```python
from build123d import *

# Parameters (mm, degrees)
BOSS_EXTRUDE1_DEPTH        = 19
F_20_0MM_DOWEL_HOLE1_D     = 24
F_20_0MM_DOWEL_HOLE1_DEPTH = 31.5
F_20_0MM_DOWEL_HOLE1_TIP   = 7.210327428


with BuildPart() as part:
    # Sketch1 → Boss-Extrude1 (new body)
    with BuildSketch(Plane(origin=(0, 0, 0), x_dir=(1, 0, 0), z_dir=(0, 1, 0))):
        Polygon((19.775, 0), (9.8875, 17.12565236), (-9.8875, 17.12565236), (-19.775, 0), (-9.8875, -17.12565236), (9.8875, -17.12565236), align=None)
    extrude(amount=BOSS_EXTRUDE1_DEPTH)

    # Sketch2 → Revolve1 (revolve)
    with BuildSketch(Plane.ZY):
        with BuildLine():
            Line((-17, 24.4), (-17, 19))
            Line((-17, 19), (0, 19))
            Line((0, 19), (0, 41.4))
            ThreePointArc((0, 41.4), (-12.02081528, 36.42081528), (-17, 24.4))
        make_face()
    revolve(axis=Axis((0, -1000, 0), (0, 1, 0)))

    # Ø20.0mm Dowel Hole1
    with Locations(Plane(origin=(0, 0, 0), x_dir=(-1, 0, 0), z_dir=(0, -1, 0))):
        with Locations((0, 0)):
            Hole(F_20_0MM_DOWEL_HOLE1_D / 2, depth=F_20_0MM_DOWEL_HOLE1_DEPTH)
            with Locations((0, 0, -(F_20_0MM_DOWEL_HOLE1_DEPTH + F_20_0MM_DOWEL_HOLE1_TIP / 2))):  # 118° drill point
                Cone(0, F_20_0MM_DOWEL_HOLE1_D / 2, F_20_0MM_DOWEL_HOLE1_TIP, mode=Mode.SUBTRACT)

    # Sketch6 → Cut-Revolve1 (revolve, cut)
    with BuildSketch(Plane.XY):
        Polygon((19.775, 19), (17, 19), (19.775, 16.225), align=None)
        Polygon((19.775, 2.775), (19.775, 0), (17, 0), align=None)
    revolve(axis=Axis((0, -1000, 0), (0, 1, 0)), mode=Mode.SUBTRACT)


solid = part.part
```
The model under review builds one solid part; all positions refer to its coordinate system, in mm. A direction names the side the tool comes from. Give positions to 0.01 mm unless a question says otherwise; leave off trailing zeros. Write each loop counter-clockwise with the first axis right and the second up, starting at its lowest first coordinate (ties: lowest second). Pieces come first, ordered by that corner, then holes. Notation, with made-up numbers: M 80,-19 L 109,-19 A19 ccw 109,1 Z; hole C 45.25,-1 d4. An arc over 180 degrees is marked long. Write item = value, one per line. Start each with the question number.
Q1. Clearance check with flat-ended pins moving along their axes: pin 1 (12 mm diameter, centred on y = 34.5, z = 2, fed in from +X); pin 2 (5 mm diameter, centred on y = 29, z = 5.5, fed in from -X); pin 3 (3 mm diameter, centred on x = -10.5, z = -4, fed in from +Y). State where each tip first meets the part, or that it passes through.
Q2. For line 1 (Z direction, x = 0, y = 7); line 2 (Z direction, x = 0, y = 23.5); line 3 (X direction, y = 23, z = -3.5), list the stretches that pass through material, from the lowest coordinate up.
Q3. We need section A-A (y = 13.5). State the section outline as (x, z) points (1 decimal).
Q4. Mouldability with a two-part tool opening along X and no side actions: class faces 1 (the face through (-14.9, 9.37, 8.44)), 2 (the face through (0, 9, 17.126)), 3 (the face through (-11.99, 15.97, -0.53)) as released by +X, released by -X, zero draft, split by the parting line, or undercut.
Q5. Machinability: for faces 4 (the face through (-0.96, 37.46, 1.85)), 5 (the face through (-14.334, 21.662, -9.139)), which of the approach directions +Z, -Z, +X, -X, +Y, -Y give a long, thin tool a straight path to every point of the face, cutting with its end or side? Answer none if there is none.
Q6. We need section B-B (y = 27). State the section outline as (x, z) points, plus the area to 3 significant figures.
Result set:
q1.pin_1 = 16.45
q1.pin_2 = -16.35
q1.pin_3 = 38.34
q2.line_1 = -17.13 to -12, 12 to 17.13
q2.line_2 = -17 to -12, 12 to 17
q2.line_3 = -16.64 to -11.48, 11.48 to 16.64
q3.outline = M -19.8,0 L -9.9,-17.1 L 9.9,-17.1 L 19.8,0 L 9.9,17.1 L -9.9,17.1 Z; hole C 0,0 d24
q4.face_1 = released by -X
q4.face_2 = zero draft
q4.face_3 = undercut
q5.face_4 = -Y
q5.face_5 = +Y
q6.outline = C 0,0 d33.6; hole C 0,0 d24
q6.area = 434 mm2
